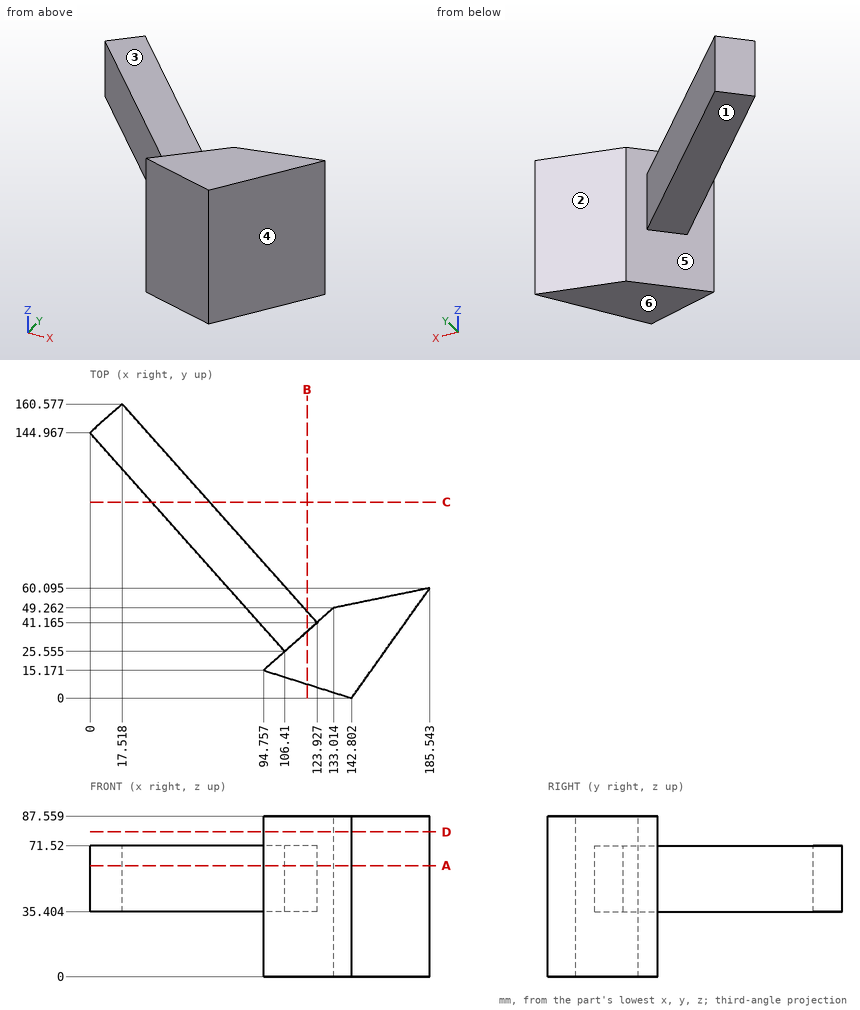
For this review, use the dimensioned drawing (mm, ordinates from the lowest corner) and the shaded views. A direction names the side the tool comes from. Give positions to 0.01 mm unless a question says otherwise; leave off trailing zeros. Loops run counter-clockwise (first coordinate to the right, second up) from the corner with the lowest first, then second, coordinate; pieces in that order, holes last.
Item 1: Take a section at D-D, the plane z = 79. State the section outline as (x, y) points (1 decimal).
Item 2: For line 1 along Z through (x, y) = (55, 97); line 2 along X through (y, z) = (41.5, 61.5) (1 decimal); line 3 along X through (y, z) = (46, 75) (1 decimal), list the stretches that pass through material, from the lowest coordinate up.
Item 3: Draft analysis for pull direction Y (two halves, no side actions). For the marked faces 4, 5 and 6, state which applies: +Y half, -Y half, draft (parallel to the pull), parting line (faces both ways), or undercut.
Item 4: Take a section at C-C, the plane y = 107. State the section outline as (x, z) points.
Item 5: Take a section at A-A, the plane z = 60.5. State the section outline as (x, y) points (1 decimal).
Item 6: Insertion check: pin 1 (8 mm diameter, centred on x = 152, z = 25.5, fed in from -Y); pin 2 (2 mm diameter, centred on y = 118.5, z = 72, fed in from -X) (1 decimal); pin 3 (2 mm diameter, centred on x = 106.5, z = 58.5, fed in from +Y) (1 decimal). Each pin has a flat end and moves straight along its axis. Give the tip position at first contact, or say it passes through.
Item 7: Tool access review of the marked faces 1, 2 and 3: name each direction out of +Z, -Z, +X, -X, +Y, -Y from which nothing blocks a thin tool from reaching the whole face with its end or side.
Item 8: Take a section at B-B, the plane x = 118.5. State the section outline as (y, z) points (1 decimal).
Calculated:
1. outline: (94.8, 15.2) - (142.8, 0) - (185.5, 60.1) - (133, 49.3) - close
2. line 1: z = 35.4 to 71.52
2. line 2: x = 92.2 to 123.6, 124.3 to 172.3
2. line 3: x = 129.4 to 175.5
3. face 4: -Y half
3. face 5: undercut
3. face 6: draft
4. outline: (33.83, 35.4) - (65.26, 35.4) - (65.26, 71.52) - (33.83, 71.52) - close
5. outline: (0, 145) - (106.4, 25.6) - (94.8, 15.2) - (142.8, 0) - (185.5, 60.1) - (133, 49.3) - (123.9, 41.2) - (17.5, 160.6) - close
6. pin 1: stops at y = 7.31
6. pin 2: stops at x = 22.8
6. pin 3: stops at y = 61.8
7. face 1: -Z, -X, +Y
7. face 2: +Z, -Z, +Y
7. face 3: +Z, -X, +Y
8. outline: (7.7, 0) - (36.3, 0) - (36.3, 35.4) - (47.3, 35.4) - (47.3, 71.5) - (36.3, 71.5) - (36.3, 87.6) - (7.7, 87.6) - close
